Part model, mm, in its own coordinate system. Give positions to 0.01 mm unless a question says otherwise; leave off trailing zeros. Write each loop counter-clockwise with the first axis right and the second up, starting at its lowest first coordinate (ties: lowest second). Pieces come first, ordered by that corner, then holes.
from build123d import *

# Parameters (mm, degrees)
SKETCH_W        = 52
SKETCH_H        = 72
PAD_DEPTH       = 2
SKETCH001_R     = 1.2
POCKET_DEPTH    = 5
SKETCH002_R     = 3.15
SKETCH002_R_2   = 1.15
PAD001_DEPTH    = 2
POCKET001_DEPTH = 5


with BuildPart() as part:
    # Sketch → Pad (new body)
    with BuildSketch(Plane.XY):
        Rectangle(SKETCH_W, SKETCH_H)
    extrude(amount=PAD_DEPTH)

    # Sketch001 (on Face6 of Pad) → Pocket (cut)
    with BuildSketch(Plane.XY.offset(2)):
        with Locations((-23, 32.95)):
            Circle(SKETCH001_R)
        with Locations((23, 32.95)):
            Circle(SKETCH001_R)
        with Locations((-23, -32.95)):
            Circle(SKETCH001_R)
        with Locations((23, -32.95)):
            Circle(SKETCH001_R)
    extrude(amount=-POCKET_DEPTH, mode=Mode.SUBTRACT)

    # Sketch002 (on Face5 of Pocket) → Pad001 (join)
    with BuildSketch(Plane.XY.offset(2)):
        with Locations((-23, 32.95)):
            Circle(SKETCH002_R)
        with Locations((-23, 32.95)):
            Circle(SKETCH002_R_2, mode=Mode.SUBTRACT)
        with Locations((23, 32.95)):
            Circle(SKETCH002_R)
        with Locations((23, 32.95)):
            Circle(SKETCH002_R_2, mode=Mode.SUBTRACT)
        with Locations((-23, -32.95)):
            Circle(SKETCH002_R)
        with Locations((-23, -32.95)):
            Circle(SKETCH002_R_2, mode=Mode.SUBTRACT)
        with Locations((23, -32.95)):
            Circle(SKETCH002_R)
        with Locations((23, -32.95)):
            Circle(SKETCH002_R_2, mode=Mode.SUBTRACT)
    extrude(amount=PAD001_DEPTH)

    # Sketch003 (on Face5 of Pad001) → Pocket001 (cut)
    with BuildSketch(Plane.XY.offset(2)):
        with BuildLine():
            Line((-18.921431, 31.109041), (18.921431, 31.109041))
            ThreePointArc((21.921431, 28.109041), (21.042751, 30.230361), (18.921431, 31.109041))
            Line((21.921431, 28.109041), (21.921431, -28.109041))
            ThreePointArc((18.921431, -31.109041), (21.042751, -30.230361), (21.921431, -28.109041))
            Line((18.921431, -31.109041), (-18.921431, -31.109041))
            ThreePointArc((-21.921431, -28.109041), (-21.042751, -30.230361), (-18.921431, -31.109041))
            Line((-21.921431, -28.109041), (-21.921431, 28.109041))
            ThreePointArc((-18.921431, 31.109041), (-21.042751, 30.230361), (-21.921431, 28.109041))
        make_face()
    extrude(amount=-POCKET001_DEPTH, mode=Mode.SUBTRACT)


solid = part.part
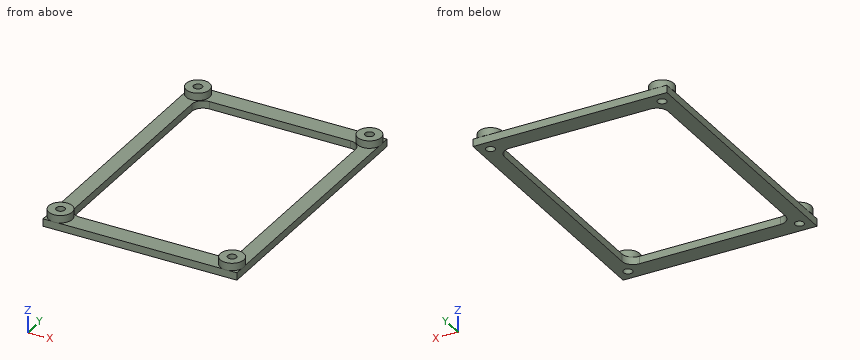
1) Drill centre lines: L1, parallel to Y at x = 23, z = 3.2; L2, parallel to Y at x = -23, z = 1.3; L3, parallel to X at y = 33, z = 3.5. Where is each one in solid material? Low to high.
Check result:
L1: y = -36.1 to -34.1, -31.8 to -29.8, 29.8 to 31.8, 34.1 to 36.1
L2: y = -36 to -34.15, -31.75 to 31.75, 34.15 to 36
L3: x = -26.15 to -24.15, -21.85 to -19.85, 19.85 to 21.85, 24.15 to 26.15
2) Flat gauge pins, fed straight in: P1, Ø1.9, axis at x = 23, y = 32.95, coming from the -Z side; P2, Ø2, axis at y = 4, z = 2, coming from the +X side; P3, Ø1.5, axis at y = 6.5, z = 1.5, coming from the -X side; P4, Ø0.6, axis at x = 6.5, z = 1.5, coming from the +Y side. Where does each tip first touch, or does it go through?
Check result:
P1: passes through
P2: stops at x = 26
P3: stops at x = -26
P4: stops at y = 36
3) Saw through at C-C (z = 0.7). Write the cut outline in (x, y).
Check result:
outline: (-26, -36) - (26, -36) - (26, 36) - (-26, 36) - close; hole circle Ø2.4 at (-23, -32.95); hole circle Ø2.4 at (-23, 32.95); hole (-21.92, -28.11) arc R3 ccw to (-18.92, -31.11) - (18.92, -31.11) arc R3 ccw to (21.92, -28.11) - (21.92, 28.11) arc R3 ccw to (18.92, 31.11) - (-18.92, 31.11) arc R3 ccw to (-21.92, 28.11) - close; hole circle Ø2.4 at (23, -32.95); hole circle Ø2.4 at (23, 32.95)
4) Saw through at B-B (x = 14). Write the cut outline in (y, z), and give its area (3 significant figures).
Check result:
outline: (-36, 0) - (-31.11, 0) - (-31.11, 2) - (-36, 2) - close; (31.11, 0) - (36, 0) - (36, 2) - (31.11, 2) - close
area: 19.6 mm2
5) Saw through at D-D (y = -13.5). Write the cut outline in (x, z).
Check result:
outline: (-26, 0) - (-21.92, 0) - (-21.92, 2) - (-26, 2) - close; (21.92, 0) - (26, 0) - (26, 2) - (21.92, 2) - close
6) Saw through at A-A (y = 32.95). Write the cut outline in (x, z).
Check result:
outline: (-26.15, 2) - (-26, 2) - (-26, 0) - (-24.2, 0) - (-24.2, 2) - (-24.15, 2) - (-24.15, 4) - (-26.15, 4) - close; (-21.85, 2) - (-21.8, 2) - (-21.8, 0) - (21.8, 0) - (21.8, 2) - (21.85, 2) - (21.85, 4) - (19.85, 4) - (19.85, 2) - (-19.85, 2) - (-19.85, 4) - (-21.85, 4) - close; (24.15, 2) - (24.2, 2) - (24.2, 0) - (26, 0) - (26, 2) - (26.15, 2) - (26.15, 4) - (24.15, 4) - close
